Can you work these out from the model? Positions are in its coordinate system, mm. A direction names the side the tool comes from. Give positions to 0.01 mm unless a question says otherwise; leave off trailing zeros. Loops run counter-clockwise (first coordinate to the right, second up) from the corner with the lowest first, then second, coordinate; pieces in that order, holes last. Notation, with made-up numbers: (5.5, 39.25) -> (39.5, 39.25) arc R21 ccw to (39.5, 78.25) -> close; hole circle Ø9 at (71.5, 27). An arc over 180 degrees is marked (long way). Return JSON: item names as keys, results as strings. Group by question number.
Q1. Suppose I cut it at D-D, the plane y = 12.5. Please give me the cut outline in (x, z).
Q2. Which directions (+Z, -Z, +X, -X, +Y, -Y) give clear straight access to the entire face, cutting with the end or side of a thin tool? Please do faces 1 (the flat face through (-5, 0, 13)), 2 (the flat face through (10, 9, 25.4)), 3 (the flat face through (-2, 9.601, 13)), 4 (the flat face through (66, 0, 13)).
Q3. I need wall thicknesses on line 1 along X through (y, z) = (12, 8.5); line 2 along Y through (x, z) = (41, 14.5); line 3 along X through (y, z) = (11.5, 11.5). Which ranges of each line are inside material? Lowest first, please. Write a range as [from, to].
Q4. Suppose I cut it at C-C, the plane z = 15.5. Please give me the cut outline in (x, y), and give its area (3 significant figures).
Q5. Thinking about a two-plate mould opening in Y: for faces 5 (the flat face through (61, 3.659, 13)), 6 (the flat face through (10, 9, 0)), 7 (the flat face through (110.86, 2.48, 12.52)), 8 (the flat face through (66, 9.601, 13)), which applies, pulls with the +Y half, pulls with the -Y half, needs draft (parallel to the pull), parting line crosses it, or undercut?
Q6. Suppose I cut it at B-B, the plane y = -2. Please give me the cut outline in (x, z).
Q7. Will these pins go through, and if not, where does the flat tip stop? pin 1 (3 mm diameter, centred on y = 13.5, z = 16.5, fed in from +X); pin 2 (10 mm diameter, centred on x = -37, z = 22.5, fed in from +Y); pin 3 (12 mm diameter, centred on y = 3.5, z = 7, fed in from -X).
Q8. Suppose I cut it at A-A, the plane x = 81. Please give me the cut outline in (y, z), and give its area (3 significant figures).
```python
from build123d import *

# Parameters (mm, degrees)
F1_DEPTH = 25.4


with BuildPart() as f1:
    # F0 (on Top) → F1 (new body)
    with BuildSketch(Plane.XY):
        Polygon((9.144, 9.6012), (4.267201, 9.6012), (-23.164801, 9.6012), (-42.9768, 20.574002), (-85.039198, 20.574002), (-94.487995, 14.478001), (-86.868003, 7.1628), (-42.367201, 7.1628), (-27.7368, 0), (-12.192, 0), (18.592801, 0), (25.2984, -9.6012), (21.945599, 0), (28.041599, -4.1148), (28.041599, 0), (32.003999, 0), (41.148003, 0), (60.655203, 0), (85.344002, 0), (104.546405, 0), (100.888811, 5.304316), (104.546405, 9.6012), (85.344002, 9.6012), (60.655203, 9.6012), (40.843204, 9.6012), (32.308798, 9.6012), (27.127199, 9.6012), (27.127199, 15.646401), (21.945599, 9.6012), (27.127199, 20.2692), (17.983202, 9.6012), align=None)
        Polygon((90.180784, 5.304316), (100.888811, 5.304316), (90.180784, 3.65947), (30.333724, 3.65947), (30.333724, 5.304316), align=None, mode=Mode.SUBTRACT)
        Polygon((117.348, 5.0292), (104.546405, 9.6012), (100.888811, 5.304316), (104.546405, 0), align=None)
    extrude(amount=F1_DEPTH)


solid = f1.part
```
Ans:
{
 "1": {"outline": "(-92.43, 0) -> (-28.4, 0) -> (-28.4, 25.4) -> (-92.43, 25.4) -> close; (20.47, 0) -> (23.35, 0) -> (23.35, 25.4) -> (20.47, 25.4) -> close; (24.43, 0) -> (27.13, 0) -> (27.13, 25.4) -> (24.43, 25.4) -> close"},
 "2": {"face 1": "+Z, -Z, -X, -Y", "face 2": "+Z, +X, -X, +Y, -Y", "face 3": "+Z, -Z, +Y", "face 4": "+Z, -Z, +X, -Y"},
 "3": {"line 1": "x = [-91.91, -27.5], [20.04, 23.11], [24, 27.13]", "line 2": "y = [0, 3.66], [5.3, 9.6]", "line 3": "x = [-91.39, -26.59], [19.61, 22.87], [23.57, 27.13]"},
 "4": {"outline": "(-94.49, 14.48) -> (-86.87, 7.16) -> (-42.37, 7.16) -> (-27.74, 0) -> (18.59, 0) -> (25.3, -9.6) -> (21.95, 0) -> (28.04, -4.11) -> (28.04, 0) -> (104.55, 0) -> (117.35, 5.03) -> (104.55, 9.6) -> (27.13, 9.6) -> (27.13, 15.65) -> (21.95, 9.6) -> (27.13, 20.27) -> (17.98, 9.6) -> (-23.16, 9.6) -> (-42.98, 20.57) -> (-85.04, 20.57) -> close; hole (30.33, 3.66) -> (90.18, 3.66) -> (100.89, 5.3) -> (30.33, 5.3) -> close", "area": "2,120 mm^2"},
 "5": {"face 5": "undercut", "face 6": "needs draft", "face 7": "pulls with the -Y half", "face 8": "pulls with the +Y half"},
 "6": {"outline": "(19.99, 0) -> (22.64, 0) -> (22.64, 25.4) -> (19.99, 25.4) -> close; (24.91, 0) -> (28.04, 0) -> (28.04, 25.4) -> (24.91, 25.4) -> close"},
 "7": {"pin 1": "stops at x = 27.13", "pin 2": "stops at y = 20.03", "pin 3": "stops at x = -89.3"},
 "8": {"outline": "(0, 0) -> (3.66, 0) -> (3.66, 25.4) -> (0, 25.4) -> close; (5.3, 0) -> (9.6, 0) -> (9.6, 25.4) -> (5.3, 25.4) -> close", "area": "202 mm^2"}
}
